Autodesk Inventor part; units mm, degrees
ref_plane "YZ Plane" through (0, 0, 0) normal (1, 0, 0) x (0, 1, 0)
ref_plane "XZ Plane" through (0, 0, 0) normal (0, 1, 0) x (-1, 0, 0)
ref_plane "XY Plane" through (0, 0, 0) normal (0, 0, 1) x (1, 0, 0)
sketch "Sketch1" plane through (0, 0, 0) normal (0, 0, 1) x (1, 0, 0)
  line L0 (0, 0) -> (80, 0)
  line L1 (0, 0) -> (0, 155)
  line L2 (80, 0) -> (80, 105)
  line L3 (80, 105) -> (0, 155)
  dimension "d0" = 80
  dimension "d1" = 155
  dimension "d2" = 105
extrude "Extrusion1" add sketch "Sketch1" along normal blind 200
sketch "Sketch3" plane through (0, 0, 200) normal (0, 0, 1) x (1, 0, 0)
  line L0 (2, 0) -> (2, 151.3915)
  line L1 (80, 0) -> (80, 105)
  line L2 (78, 0) -> (78, 103.8915)
  line L3 (80, 105) -> (0, 155)
  line L4 (2, 151.3915) -> (78, 103.8915)
  line L5 (0, 0) -> (80, 0)
  line L6 (2, 0) -> (78, 0)
  line L7 (0, 155) -> (0, 0)
  dimension "d23" = 2
  dimension "d24" = 2
  dimension "d25" = 2
extrude "Extrusion3" cut sketch "Sketch3" against normal blind 197 contours L0 L4 L2 L5
extrude "Extrusion4" add sketch "Sketch3" against normal blind 3 contours L0 L4 L2 L5
sketch "Sketch4" plane through (0, 0, 0) normal (-1, 0, 0) x (0, 0, 1)
  line L0 (0, 155) -> (0, 0)
  line L1 (0, 155) -> (0, 105)
  line L2 (28, 99.083) -> (42, 99.083)
  line L3 (42, 99.083) -> (42, 104)
  line L4 (42, 104) -> (28, 104)
  line L5 (28, 104) -> (28, 99.083)
  line L6 (28, 99.083) -> (42, 99.083)
  line L7 (0, 155) -> (0, 105)
  line L8 (0, 155) -> (200, 155)
  line L9 (28, 99.083) -> (42, 99.083)
  point P0 (28, 101.5415)
  dimension "d47" = 28
  dimension "d48" = 51
extrude "Extrusion5" cut sketch "Sketch4" against normal blind 10
sketch "Sketch5" plane through (2, 0, 3) normal (1, 0, 0) x (0, 0, -1)
  line L0 (-25, 99.083) -> (-39, 99.083)
  line L1 (-25, 99.083) -> (-22, 99.083)
  line L2 (-39, 99.083) -> (-42, 99.083)
  line L3 (-42, 99.083) -> (-22, 99.083)
  line L4 (-22, 99.083) -> (-22, 96.083)
  line L5 (-22, 96.083) -> (-42, 96.083)
  line L6 (-42, 96.083) -> (-42, 99.083)
  point P0 (3, 0)
  dimension "d42" = 3
  dimension "d43" = 3
  dimension "d44" = 3
extrude "Extrusion6" add sketch "Sketch5" along normal blind 60
sketch "Sketch6" plane through (0, 155, 200) normal (0.53, 0.848, 0) x (0.848, -0.53, 0)
  line L0 (25, 15) -> (50.5, 15)
  line L1 (50.5, 15) -> (50.5, 85.5)
  line L2 (50.5, 85.5) -> (25, 85.5)
  line L3 (25, 85.5) -> (25, 15)
  line L4 (94.3398, 0) -> (0, 0)
  line L5 (0, 200) -> (0, 0)
  line L6 (32.9219, 175) -> (83.8018, 175)
  circle A0 centre (37.75, 175) radius 7.75
  circle A1 centre (37.75, 134.2821) radius 7.75
  line L7 (82.3488, 140) -> (57.3488, 140)
  line L8 (57.3488, 140) -> (57.3488, 170)
  line L9 (57.3488, 170) -> (82.3488, 170)
  line L10 (82.3488, 170) -> (82.3488, 140)
  line L11 (31.3319, 155) -> (82.2118, 155)
  line L12 (82.3488, 140) -> (57.3488, 170) construction
  line L13 (57.3488, 140) -> (82.3488, 170) construction
  point P0 (82.1498, 200)
  point P1 (69.8488, 155)
  dimension "d49" = 25.5
  dimension "d50" = 70.5
  dimension "d51" = 15
  dimension "d52" = 25
  dimension "d53" = 15.5
  dimension "d54" = 15.5
  dimension "d55" = 25
  dimension "d56" = 30
extrude "Extrusion7" cut sketch "Sketch6" against normal blind 10
properties part number "Housing og Buttons & LCD"
Part model, mm, in its own coordinate system. A direction names the side the tool comes from. Coordinates: 2 decimals unless noted, no trailing zeros. Order: outer loops, then holes, each group sorted by start corner. A loop starts at its lowest first (then second) coordinate and runs counter-clockwise, first axis right, second up. Notation, with made-up numbers: (78, 78) - (108, 78) arc R21 cw to (108, 114) - close; hole circle Ø9 at (13.5, 42.5). An arc over 180 degrees is marked (long way). Use CSV: the item, a comma, the result in double quotes.
Item 1: Probe probe 1 along Z at (x, y) = (55, 58); probe 2 along X at (y, z) = (77.5, 52); probe 3 along X at (y, z) = (140, 179.5). List the from-to ranges inside material, lowest first.
Solved:
probe 1,"z = 0 to 3, 197 to 200"
probe 2,"x = 0 to 2, 78 to 80"
probe 3,"x = 0 to 2"
Item 2: Drop flat-ended pins along their axis: P1, Ø8, axis at x = 34, z = 109, coming from the -Y side; P2, Ø22, axis at x = 42.5, z = 31, coming from the +Y side; P3, Ø1, axis at x = 28, z = 46.5, coming from the +Y side. Give the stop position or say it passes through.
Solved:
P1,"stops at y = 128.89"
P2,"stops at y = 135.23"
P3,"stops at y = 137.81"
Item 3: 3-axis set-ups, long thin cutter, end or side, ignore diameter. For faces 4 (the face through (39, 60, 3)), 5 (the face through (30.065, 135.047, 73.284)): which of +Z, -Z, +X, -X, +Y, -Y reach the whole face in a straight line?
Solved:
face 4,"-Y"
face 5,"none"
Item 4: Saw through at D-D on z = 100. Give the cut face in (x, y), and give its area (3 significant figures).
Solved:
outline,"(0, 0) - (2, 0) - (2, 151.39) - (78, 103.89) - (78, 0) - (80, 0) - (80, 105) - (0, 155) - close"
area,"699 mm²"
Item 5: Saw through at A-A on z = 158. Give the cut face in (x, y).
Solved:
outline,"(0, 0) - (2, 0) - (2, 151.39) - (20.14, 140.05) - (21.2, 141.75) - (0, 155) - close; (41.76, 126.54) - (78, 103.89) - (78, 0) - (80, 0) - (80, 105) - (42.82, 128.24) - close"
Item 6: Saw through at B-B on y = 25. Give the cut face in (x, z), and give its area (3 significant figures).
Solved:
outline,"(0, 0) - (80, 0) - (80, 200) - (0, 200) - close; hole (2, 3) - (78, 3) - (78, 197) - (2, 197) - close"
area,"1,260 mm²"
Item 7: Mould opens along X. For faces 1 (the face through (1, 0, 100)), 2 (the face through (80, 52, 99)), 3 (the face through (31, 99.083, 35)) say: +X half, -X half, draft (parallel to the pull), parting line (faces both ways), or undercut.
Solved:
face 1,"draft"
face 2,"+X half"
face 3,"undercut"
Item 8: Saw through at C-C on x = 57. Give the cut face in (y, z) (1 decimal).
Solved:
outline,"(0, 0) - (119.4, 0) - (119.4, 30) - (117, 30) - (117, 3) - (0, 3) - close; (0, 197) - (117, 197) - (117, 60) - (119.4, 60) - (119.4, 200) - (0, 200) - close; (96.1, 25) - (99.1, 25) - (99.1, 45) - (96.1, 45) - close"
